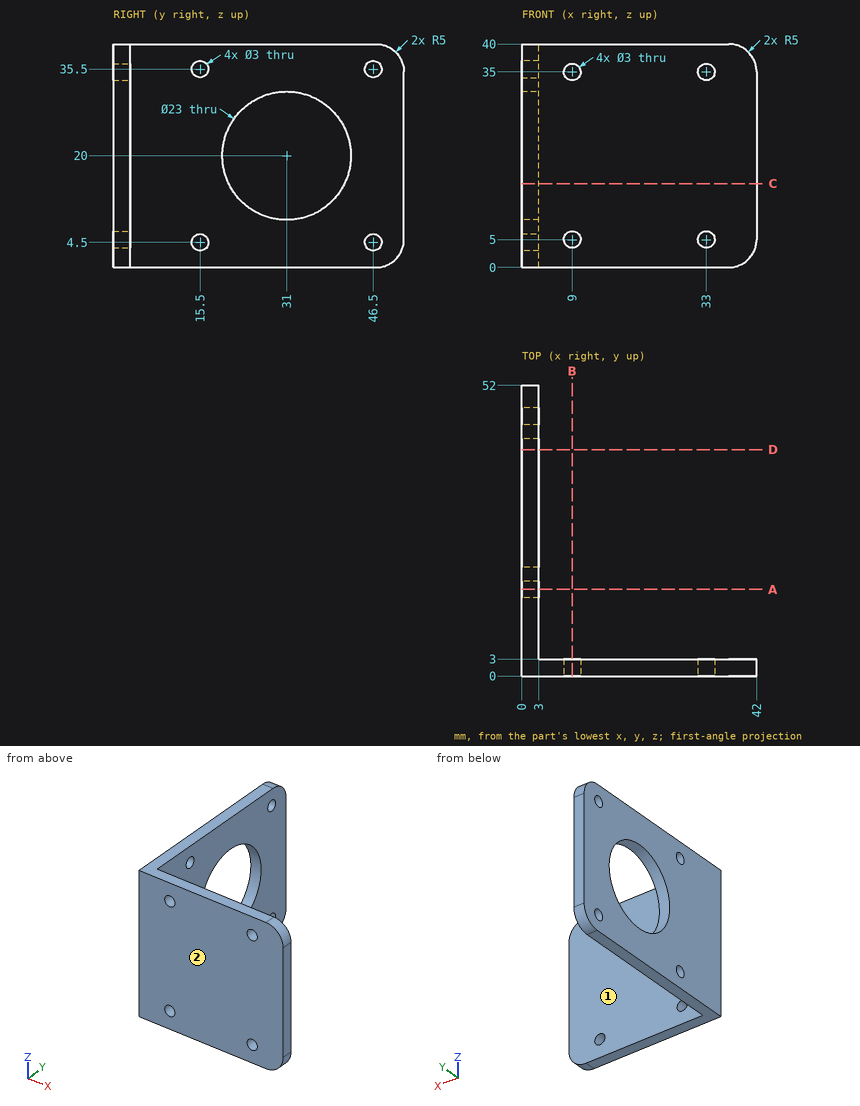
Can you work these out from the drawing? Everything is in mm from the part's minimum corner. A direction names the side the tool comes from. Give positions to 0.01 mm unless a question says otherwise; leave off trailing zeros. Order: outer loops, then holes, each group sorted by start corner. A loop starts at its lowest first (then second) coordinate and runs counter-clockwise, first axis right, second up.
1. Suppose I cut it at C-C (z = 15). List the corners of the cut face in (x, y) for me, plus the area to 3 significant figures.
2. Suppose I cut it at A-A (y = 15.5). List the corners of the cut face in (x, z) for me, plus the area to 3 significant figures.
3. For the marked faces 1 and 2, which set-ups out of +Z, -Z, +X, -X, +Y, -Y let a thin tool reach every point of the face, with its end or its side?
4. Will these pins go through, and if not, where does the flat tip stop? P1, Ø20, axis at y = 32.5, z = 11, coming from the +X side; P2, Ø3.5, axis at x = 33, z = 5, coming from the +Y side.
5. Suppose I cut it at D-D (y = 40.5). List the corners of the cut face in (x, z) for me, plus the area to 3 significant figures.
6. I need wall thicknesses on L1, parallel to X at y = 1.8, z = 5; L2, parallel to Y at x = 1.45, z = 4.5; L3, parallel to Z at x = 1, y = 15. Which ranges of each line are inside material? Lowest first, please.
7. Suppose I cut it at B-B (x = 9). List the corners of the cut face in (y, z) for me, plus the area to 3 significant figures.
Solved:
1. outline: (0, 0) - (42, 0) - (42, 3) - (3, 3) - (3, 20.64) - (0, 20.64) - close; (0, 41.36) - (3, 41.36) - (3, 52) - (0, 52) - close
1. area: 211 mm2
2. outline: (0, 0) - (3, 0) - (3, 3) - (0, 3) - close; (0, 6) - (3, 6) - (3, 34) - (0, 34) - close; (0, 37) - (3, 37) - (3, 40) - (0, 40) - close
2. area: 102 mm2
3. face 1: +Z, -Z, +X, +Y
3. face 2: +Z, -Z, +X, -X, -Y
4. P1: stops at x = 3
4. P2: stops at y = 3
5. outline: (0, 0) - (3, 0) - (3, 13.52) - (0, 13.52) - close; (0, 26.48) - (3, 26.48) - (3, 40) - (0, 40) - close
5. area: 81.1 mm2
6. L1: x = 0 to 7.5, 10.5 to 31.5, 34.5 to 42
6. L2: y = 0 to 14, 17 to 45, 48 to 51.97
6. L3: z = 0 to 3.09, 5.91 to 34.09, 36.91 to 40
7. outline: (0, 0) - (3, 0) - (3, 3.5) - (0, 3.5) - close; (0, 6.5) - (3, 6.5) - (3, 33.5) - (0, 33.5) - close; (0, 36.5) - (3, 36.5) - (3, 40) - (0, 40) - close
7. area: 102 mm2
